Autodesk Inventor part; units mm, degrees
ref_plane "YZ Plane" through (0, 0, 0) normal (1, 0, 0) x (0, 1, 0)
ref_plane "XZ Plane" through (0, 0, 0) normal (0, 1, 0) x (-1, 0, 0)
ref_plane "XY Plane" through (0, 0, 0) normal (0, 0, 1) x (1, 0, 0)
sketch "Boceto1" plane through (0, 0, 0) normal (0, 1, 0) x (-1, 0, 0)
  line L0 (-80, 120) -> (80, 120)
  line L1 (80, 120) -> (80, -120)
  line L2 (80, -120) -> (-80, -120)
  line L3 (-80, -120) -> (-80, 120)
  line L4 (-80, 120) -> (80, -120) construction
  line L5 (80, 120) -> (-80, -120) construction
  point P0 (0, 0)
  dimension "d0" = 160
  dimension "d1" = 240
extrude "Extrusión1" add sketch "Boceto1" along normal blind 10
sketch "Boceto2" plane through (0, 10, 0) normal (0, 1, 0) x (1, 0, 0)
  line L0 (-80, -120) -> (80, -120)
  line L1 (80, -120) -> (80, 120)
  line L2 (80, 120) -> (-80, 120)
  line L3 (-80, 120) -> (-80, -120)
  line L4 (-75, 115) -> (75, 115) construction
  line L5 (75, 115) -> (75, -115) construction
  line L6 (75, -115) -> (-75, -115) construction
  line L7 (-75, -115) -> (-75, 115) construction
  point P0 (0, 0)
  point P1 (-75, 0)
  point P2 (75, 0)
  point P3 (0, -115)
  point P4 (0, 115)
  dimension "d4" = 5
hole "Agujero1" at (-75, 10, 0) at (75, 10, 0) at (0, 10, 115) at (0, 10, -115) at (-75, 10, -115) at (75, 10, -115) at (75, 10, 115) at (-75, 10, 115) direction (0, -1, 0) diameter 8 depth 15 tip angle 118
properties part number "TAPA SUPERIOR" material "Plástico PMMA"
The listing builds one solid part. Answer for the finished solid, in the listing's coordinates (mm). Round coordinates to 2 decimals unless told otherwise and drop trailing zeros. Loops run counter-clockwise (first coordinate to the right, second up) from the corner with the lowest first, then second, coordinate; pieces in that order, holes last.
Q1. Find the intervals of material crossed by line 1 (Z direction, x = 75, y = 6.75); line 2 (X direction, y = 5.25, z = -115); line 3 (Z direction, x = 0, y = 5.75), in increasing order.
Q2. Section B-B, the plane z = 0 is taken. Determine the outline of the cut face in (x, y), then the cut area to 3 significant figures.
Q3. Section A-A, the plane x = 0 is taken. Determine the outline of the cut face in (y, z).
Q4. Section D-D, the plane z = 115 is taken. Determine the outline of the cut face in (x, y).
Q5. Section C-C, the plane x = -75 is taken. Determine the outline of the cut face in (y, z).
Q6. For a pull along Z with two mould halves and no side action, classify faces 1 (the face through (1, 5, 120)), 2 (the face through (78.905, 4.93, -0.867)), 3 (the face through (-80, 5, 2)) as released by +Z, released by -Z, zero draft, split by the parting line, or undercut.
Completed:
1. line 1: z = -120 to -119, -111 to -4, 4 to 111, 119 to 120
1. line 2: x = -80 to -79, -71 to -4, 4 to 71, 79 to 80
1. line 3: z = -120 to -119, -111 to 111, 119 to 120
2. outline: (-80, 0) - (-79, 0) - (-79, 10) - (-80, 10) - close; (-71, 0) - (71, 0) - (71, 10) - (-71, 10) - close; (79, 0) - (80, 0) - (80, 10) - (79, 10) - close
2. area: 1,440 mm2
3. outline: (0, -120) - (10, -120) - (10, -119) - (0, -119) - close; (0, -111) - (10, -111) - (10, 111) - (0, 111) - close; (0, 119) - (10, 119) - (10, 120) - (0, 120) - close
4. outline: (-80, 0) - (-79, 0) - (-79, 10) - (-80, 10) - close; (-71, 0) - (-4, 0) - (-4, 10) - (-71, 10) - close; (4, 0) - (71, 0) - (71, 10) - (4, 10) - close; (79, 0) - (80, 0) - (80, 10) - (79, 10) - close
5. outline: (0, -120) - (10, -120) - (10, -119) - (0, -119) - close; (0, -111) - (10, -111) - (10, -4) - (0, -4) - close; (0, 4) - (10, 4) - (10, 111) - (0, 111) - close; (0, 119) - (10, 119) - (10, 120) - (0, 120) - close
6. face 1: released by +Z
6. face 2: undercut
6. face 3: zero draft
